Autodesk Inventor part; units mm, degrees
ref_plane "Work Plane1" through (0, -40, 0) normal (1, 0, 0) x (0, 0, -1)
ref_plane "Work Plane2" through (0, 0, 90) normal (0, 0, 1) x (1, 0, 0)
ref_plane "YZ Plane" through (0, 0, 0) normal (1, 0, 0) x (0, 1, 0)
sketch "Sketch5" plane through (0, 0, 0) normal (0, 0, 1) x (1, 0, 0)
  line L0 (-12.5, 10) -> (12.5, 10)
  line L1 (12.5, 10) -> (12.5, -40)
  line L2 (12.5, -40) -> (-12.5, -40)
  line L3 (-12.5, -40) -> (-12.5, 10)
  circle A0 centre (0, 0) radius 7.5
  dimension "d11" = 25
  dimension "d12" = 50
  dimension "d13" = 15
  dimension "d14" = 10
  dimension "d15" = 12.5
extrude "Extrusion4" add sketch "Sketch5" along normal blind 10
sketch "Sketch6" plane through (0, 0, 10) normal (0, 0, 1) x (1, 0, 0)
  circle A0 centre (0, 0) radius 7.5
  line L0 (-7.5, 0) -> (-12.5, 0)
  line L1 (-12.5, 10) -> (-12.5, -40)
  line L2 (-12.5, 10) -> (-12.5, 0)
  line L3 (12.5, 10) -> (-12.5, 10)
  line L4 (12.5, -40) -> (12.5, 10)
  line L5 (-12.5, 10) -> (12.5, 10)
  line L6 (12.5, 10) -> (12.5, 0)
  line L7 (12.5, 0) -> (7.5, 0)
  arc A1 (7.5, 0) -> (-7.5, 0) centre (0, 0) ccw
extrude "Extrusion5" add sketch "Sketch6" along normal blind 15 contours A0 L0 L1 L3 L4 L7
sketch "Sketch7" plane through (0, 0, 25) normal (0, 0, 1) x (1, 0, 0)
  line L0 (-12.5, 10) -> (-12.5, -40)
  line L1 (12.5, -40) -> (12.5, 0)
  line L2 (-12.5, 10) -> (12.5, 10)
  line L3 (12.5, 10) -> (12.5, -20)
  line L4 (12.5, -20) -> (-12.5, -20)
  line L5 (-12.5, -20) -> (-12.5, 10)
  point P0 (0, 0)
  point P1 (-12.5, -20)
  point P2 (12.5, 0)
  dimension "d20" = 30
extrude "Extrusion6" add sketch "Sketch7" along normal blind 10
ref_plane "Work Plane1" through (0, -40, 0) normal (1, 0, 0) x (0, 0, -1)
ref_plane "Work Plane2" through (0, 0, 90) normal (0, 0, 1) x (1, 0, 0)
sketch "Sketch12" plane through (0, 0, 90) normal (0, 0, 1) x (1, 0, 0)
  line L0 (0, 28.6) -> (0, -101.6)
  line L1 (-23.1, 0) -> (51.1, 0)
  arc A0 (20.5, -66) -> (35.5, -66) centre (28, -66) ccw
  line L2 (20.5, -66) -> (15.5, -66)
  line L3 (15.5, -66) -> (15.5, -83)
  line L4 (15.5, -83) -> (40.5, -83)
  line L5 (40.5, -83) -> (40.5, -66)
  line L6 (40.5, -66) -> (35.5, -66)
  point P0 (0, 0)
  dimension "d55" = 15
  dimension "d56" = 5
  dimension "d57" = 17
  dimension "d58" = 25
sketch "Sketch13" plane through (0, 0, 10) normal (0, 0, 1) x (1, 0, 0)
  line L0 (-7.5, -23) -> (-12.5, -23)
  line L1 (-12.5, 0) -> (-12.5, -40)
  line L2 (-12.5, -23) -> (-12.5, -40)
  line L3 (-12.5, -40) -> (12.5, -40)
  line L4 (-12.5, -40) -> (12.5, -40)
  line L5 (12.5, -40) -> (12.5, -23)
  line L6 (12.5, -40) -> (12.5, 0)
  line L7 (12.5, -23) -> (7.5, -23)
  arc A0 (-7.5, -23) -> (7.5, -23) centre (0, -23) ccw
  line L8 (-12.5, -31.5) -> (12.5, -31.5)
  point P0 (0, 0)
  dimension "d48" = 5
  dimension "d49" = 5
  dimension "d50" = 7.5
  dimension "d51" = 17
sketch "Sketch14" plane through (0, 0, 0) normal (1, 0, 0) x (0, 1, 0)
  line L0 (-40, 10) -> (0, 10)
  line L1 (-40, 0) -> (-40, 10)
  line L2 (-31.5, 10) -> (-38.7794, 30)
  point P0 (0, 0)
  dimension "d62" = 8.5
  dimension "d63" = 70
  dimension "d64" = 20
sweep "Sweep2" add profiles "Sketch13" path "Sketch14" path curves L2
loft "Loft1" add profiles "Sketch12" section 1 edges at (0, -47.2794, 30) (12.5, -38.7794, 30) (10, -30.2794, 30) (0, -37.7794, 30) (-10, -30.2794, 30) (-12.5, -38.7794, 30)
sketch "Sketch15" plane through (15.5, -83, 90) normal (0, 0, 1) x (1, 0, 0)
  line L0 (5, 17) -> (-23, 52.7206)
  line L1 (0, 17) -> (5, 17)
  line L2 (5, 17) -> (0, 17)
  line L3 (0, 0) -> (0, 17)
  line L4 (0, 17) -> (0, 0)
  line L5 (25, 0) -> (0, 0)
  line L6 (0, 0) -> (25, 0)
  line L7 (25, 17) -> (25, 0)
  line L8 (25, 0) -> (25, 17)
  line L9 (20, 17) -> (25, 17)
  line L10 (25, 17) -> (20, 17)
  arc A0 (5, 17) -> (20, 17) centre (12.5, 17) ccw
  point P0 (-15.5, 83)
extrude "Extrusion7" add sketch "Sketch15" along normal blind 10
properties part number "ramp(2)"
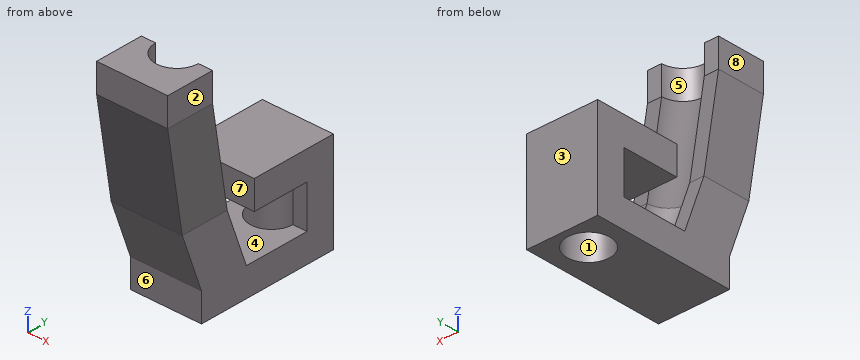
CAD build for the part. Positions are in the model's coordinates, mm. Face numbers are marked on the shaded views. A direction names the side the tool comes from. Round coordinates to 2 decimals unless told otherwise and drop trailing zeros. Write each loop counter-clockwise with the first axis right and the second up, starting at its lowest first coordinate (ties: lowest second). Pieces come first, ordered by that corner, then holes. Notation, with made-up numbers: (9.5, -34) - (25.5, -34) arc R20 ccw to (25.5, -6) - close; hole circle Ø7 at (-19, -35). An arc over 180 degrees is marked (long way). Write item = value, one per line. Start each with the question number.
Q1. Which spindle directions (+Z, -Z, +X, -X, +Y, -Y) get a long thin tool onto all of the face, cutting with end or side? Do the marked faces 4, 5, 6, 7 and 8. Say none if no direction does.
Q2. Probe L1, parallel to X at y = 0, z = 6; L2, parallel to Y at x = 0, z = 6; L3, parallel to Z at x = -6, y = -19.5. List the from-to ranges inside material, lowest first. Write a range as from..to.
Q3. Mould opens along Y. For the marked faces 1, 2 and 3 say: pulls with the +Y half, pulls with the -Y half, needs draft (parallel to the pull), parting line crosses it, or undercut.
Q4. Band-saw the part on A-A (y = -4.5). Give the cut face in (x, z), then the cut area to 3 significant figures.
Q5. Drop flat-ended pins along their axis: pin 1 (12.5 mm diameter, centred on x = 5.5, y = -12, fed in from +Z); pin 2 (1 mm diameter, centred on x = 4.5, y = -68.5, fed in from -Z); pin 3 (5 mm diameter, centred on x = -3.5, z = 30, fed in from -Y). Give the stop position or say it passes through.
Answers below:
q1.face_4 = none
q1.face_5 = +Z, +Y
q1.face_6 = -Z, +X, -X, -Y
q1.face_7 = +Z, +X, -X
q1.face_8 = +Z, -X, +Y, -Y
q2.L1 = -12.5..-7.5, 7.5..12.5
q2.L2 = -40..-7.5, 7.5..10
q2.L3 = 0..10, 25..35
q3.face_1 = undercut
q3.face_2 = needs draft
q3.face_3 = pulls with the +Y half
q4.outline = (-12.5, 0) - (-6, 0) - (-6, 10) - (-12.5, 10) - close; (-12.5, 25) - (12.5, 25) - (12.5, 35) - (-12.5, 35) - close; (6, 0) - (12.5, 0) - (12.5, 10) - (6, 10) - close
q4.area = 380 mm2
q5.pin_1 = 35
q5.pin_2 = 64.8
q5.pin_3 = -48.77
